CAD build for the part. Positions are in the model's coordinates, mm. A direction names the side the tool comes from. Give positions to 0.01 mm unless a question says otherwise; leave off trailing zeros. Loops run counter-clockwise (first coordinate to the right, second up) from the corner with the lowest first, then second, coordinate; pieces in that order, holes last. Notation, with made-up numbers: M 44,28 L 103,28 A22 cw 103,37 Z; hole C 43,-38 d9. An arc over 180 degrees is marked long. One line per question, with ' | ' between items.
Autodesk Fusion 360 part; units mm, degrees
sketch "Sketch1" plane through (0, 0, 0) normal (0, 0, 1) x (1, 0, 0)
  line L0 (37.5, 12.5) -> (-37.5, 12.5)
  line L1 (-37.5, 12.5) -> (-37.5, -12.5)
  line L2 (-37.5, -12.5) -> (37.5, -12.5)
  line L3 (37.5, -12.5) -> (37.5, 12.5)
  line L4 (37.5, 12.5) -> (-37.5, -12.5) construction
  line L5 (-37.5, 12.5) -> (37.5, -12.5) construction
  line L6 (-40, -15) -> (40, -15)
  line L7 (40, -15) -> (40, 15)
  line L8 (40, 15) -> (-40, 15)
  line L9 (-40, 15) -> (-40, -15)
  line L10 (-34.5, -9.5) -> (34.5, -9.5)
  line L11 (34.5, -9.5) -> (34.5, 9.5)
  line L12 (34.5, 9.5) -> (-34.5, 9.5)
  line L13 (-34.5, 9.5) -> (-34.5, -9.5)
  line L14 (0, 15) -> (0, -15)
  circle A0 centre (-32.5, 7.5) radius 0.75
  circle A1 centre (-32.5, 7.5) radius 2
  circle A2 centre (-32.5, -7.5) radius 2
  circle A3 centre (-32.5, -7.5) radius 0.75
  circle A4 centre (32.5, -7.5) radius 0.75
  circle A5 centre (32.5, -7.5) radius 2
  circle A6 centre (32.5, 7.5) radius 0.75
  circle A7 centre (32.5, 7.5) radius 2
  line L15 (-32.5, 7.5) -> (-28.1699, 0)
  line L16 (-28.1699, 0) -> (-32.5, -7.5)
  line L17 (32.5, -7.5) -> (28.1699, 0)
  line L18 (28.1699, 0) -> (32.5, 7.5)
  dimension "d1" = 75
  dimension "d2" = 25
  dimension "d3" = 2.5
  dimension "d4" = -3
  dimension "d5" = 1.5
  dimension "d6" = 4
  dimension "d7" = 4
  dimension "d8" = 1.5
  dimension "d9" = 1.5
  dimension "d10" = 4
  dimension "d11" = 1.5
  dimension "d12" = 4
  dimension "d16" = 30
  dimension "d17" = 30
  dimension "d18" = 30
  dimension "d19" = 30
extrude "Extrude1" add sketch "Sketch1" against normal blind 3 contours L0 L2 L3 L10 L11 L12 L14 | L0 L2 L3 L6 L7 L8 L14 | L0 L1 L2 L10 L12 L13 L14 | L0 L1 L2 L6 L8 L9 L14 | L10 L12 L14 A1 A2 L15 L16 | L10 L12 L14 A5 A7 L17 L18 | L11 L12 A7 | A6 | A7 | L12 L13 A1 | A0 | A1 | L11 A5 A7 L17 L18 | L13 A1 A2 L15 L16 | L10 L13 A2 | A3 | A2 | L10 L11 A5 | A4 | A5
extrude "Extrude2" add sketch "Sketch1" along normal blind 4 contours L0 L2 L3 L6 L7 L8 L14 | L0 L1 L2 L6 L8 L9 L14
extrude "Extrude3" add sketch "Sketch1" along normal blind 2.5 contours A6 | A7 | A0 | A1 | A3 | A2 | A4 | A5
extrude "Extrude5" add sketch "Sketch1" along normal blind 5 contours A6 | A0 | A3 | A4
Item 1: Drop a flat-ended pin along its axis: P1, Ø5, axis at x = 17.5, y = -6.5, coming from the +Z side. Give the stop position or say it passes through.
Conclusion:
P1: z = 0
Item 2: Saw through at B-B on y = 0.5. Give the cut face in (x, z), and give its area (3 significant figures).
Conclusion:
outline: M -40,-3 L 40,-3 L 40,4 L 37.5,4 L 37.5,0 L -37.5,0 L -37.5,4 L -40,4 Z | area: 260 mm²
Item 3: Saw through at A-A on z = 1.5. Give the cut face in (x, y).
Conclusion:
outline: M -40,-15 L 40,-15 L 40,15 L -40,15 Z; C -32.5,-7.5 d4; C -32.5,7.5 d4; C 32.5,-7.5 d4; C 32.5,7.5 d4; hole M -37.5,-12.5 L 37.5,-12.5 L 37.5,12.5 L -37.5,12.5 Z
Item 4: 3-axis set-ups, long thin cutter, end or side, ignore diameter. For faces 1 (the flat face through (-1, 0, 0)), 2 (the flat face through (32.5, -7.5, 5)): which of +Z, -Z, +X, -X, +Y, -Y reach the whole face in a straight line?
Conclusion:
face 1: +Z | face 2: +Z, +X, -X, +Y, -Y
Item 5: Saw through at D-D on y = 7.5. Give the cut face in (x, z), and give its area (4 significant figures).
Conclusion:
outline: M -40,-3 L 40,-3 L 40,4 L 37.5,4 L 37.5,0 L 34.5,0 L 34.5,2.5 L 33.25,2.5 L 33.25,5 L 31.75,5 L 31.75,2.5 L 30.5,2.5 L 30.5,0 L -30.5,0 L -30.5,2.5 L -31.75,2.5 L -31.75,5 L -33.25,5 L -33.25,2.5 L -34.5,2.5 L -34.5,0 L -37.5,0 L -37.5,4 L -40,4 Z | area: 287.5 mm²
Item 6: Saw through at C-C on x = -18.5. Give the cut face in (y, z).
Conclusion:
outline: M -15,-3 L 15,-3 L 15,4 L 12.5,4 L 12.5,0 L -12.5,0 L -12.5,4 L -15,4 Z
Item 7: Drill centre lines: line 1 along X through (y, z) = (8.75, 3.25); line 2 along Y through (x, z) = (-17, 1.25); line 3 along Z through (x, y) = (-5.5, -4.5). Where is each one in solid material? Low to high. Write a range as [from, to].
Conclusion:
line 1: [-40, -37.5], [37.5, 40] | line 2: [-15, -12.5], [12.5, 15] | line 3: [-3, 0]
Item 8: Mould opens along X. For faces 3 (the flat face through (-1, -15, 0)), 4 (the cylindrical face through (-31.785, -7.725, 3.732)) say: pulls with the +X half, pulls with the -X half, needs draft (parallel to the pull), parting line crosses it, or undercut.
Conclusion:
face 3: needs draft | face 4: undercut
